```python
from build123d import *

# Parameters (mm, degrees)
EXTRUDE_1_DEPTH          = 129
CUT_EXTRUDE_1_DEPTH      = 131.732551417
CUT_EXTRUDE_1_DEPTH_BACK = 131.732551417
SKETCH_2_R               = 2.5
SKETCH_2_R_2             = 2


with BuildPart() as part:
    # 草图1 → 凸台-拉伸1 (new, symmetric)
    with BuildSketch(Plane(origin=(0, 0, 0), x_dir=(0, 0, -1), z_dir=(1, 0, 0))):
        with BuildLine():
            Line((-11, -15), (11, -15))
            ThreePointArc((11, -15), (13.828427125, -13.828427125), (15, -11))
            Line((15, -11), (15, 11))
            ThreePointArc((15, 11), (13.828427125, 13.828427125), (11, 15))
            Line((11, 15), (-11, 15))
            ThreePointArc((-11, 15), (-13.828427125, 13.828427125), (-15, 11))
            Line((-15, 11), (-15, -11))
            ThreePointArc((-15, -11), (-13.828427125, -13.828427125), (-11, -15))
        make_face()
        with BuildLine():
            Line((-11, -13), (11, -13))
            ThreePointArc((11, -13), (12.414213562, -12.414213562), (13, -11))
            Line((13, -11), (13, 11))
            ThreePointArc((13, 11), (12.414213562, 12.414213562), (11, 13))
            Line((11, 13), (-11, 13))
            ThreePointArc((-11, 13), (-12.414213562, 12.414213562), (-13, 11))
            Line((-13, 11), (-13, -11))
            ThreePointArc((-13, -11), (-12.414213562, -12.414213562), (-11, -13))
        make_face(mode=Mode.SUBTRACT)
    extrude(amount=EXTRUDE_1_DEPTH, both=True)

    # 草图2 → 切除-拉伸1 (cut, two sides: drawn at the far end of the back side and taken through both)
    with BuildSketch(Plane.XY.offset(-CUT_EXTRUDE_1_DEPTH_BACK)):
        with Locations((-75, -2.5)):
            Circle(SKETCH_2_R)
        with Locations(Location((75, -2.5, 0), (0, 0, 90))):
            Circle(SKETCH_2_R)
        with Locations((-65, -2.5)):
            Circle(SKETCH_2_R_2)
        with Locations(Location((65, -2.5, 0), (0, 0, 90))):
            Circle(SKETCH_2_R_2)
    extrude(amount=CUT_EXTRUDE_1_DEPTH + CUT_EXTRUDE_1_DEPTH_BACK, mode=Mode.SUBTRACT)


solid = part.part
```
Here's how the part is built. I have some questions about the finished solid (model axes, mm). A direction names the side the tool comes from. Give positions to 0.01 mm unless a question says otherwise; leave off trailing zeros. Loops run counter-clockwise (first coordinate to the right, second up) from the corner with the lowest first, then second, coordinate; pieces in that order, holes last. Notation, with made-up numbers: M -16,61 L -10,61 A20 ccw -10,80 Z; hole C -18.75,-23 d9. An arc over 180 degrees is marked long. Return JSON: item names as keys, results as strings.
Item 1: Thinking about a two-plate mould opening in X: for faces 3 (the flat face through (129, 0, 14)), 4 (the cylindrical face through (77, -1, 14)), 5 (the cylindrical face through (1.806, -13.797, 13.859)), which applies, released by +X, released by -X, zero draft, split by the parting line, or undercut?
A:
{"face 3": "released by +X", "face 4": "undercut", "face 5": "zero draft"}
Item 2: Imagine slicing it at A-A on x = 75. List the corners of the cut face in (y, z) for me.
A:
{"outline": "M -15,-11 A4 ccw -11,-15 L -5,-15 L -5,-13 L -11,-13 A2 cw -13,-11 L -13,11 A2 cw -11,13 L -5,13 L -5,15 L -11,15 A4 ccw -15,11 Z; M 0,-15 L 11,-15 A4 ccw 15,-11 L 15,11 A4 ccw 11,15 L 0,15 L 0,13 L 11,13 A2 cw 13,11 L 13,-11 A2 cw 11,-13 L 0,-13 Z"}
Item 3: Imagine slicing it at B-B on y = 6.5. List the corners of the cut face in (x, z) for me.
A:
{"outline": "M -129,-15 L 129,-15 L 129,-13 L -129,-13 Z; M -129,13 L 129,13 L 129,15 L -129,15 Z"}
Item 4: Imagine slicing it at D-D on x = 8.5. List the corners of the cut face in (y, z) for me.
A:
{"outline": "M -15,-11 A4 ccw -11,-15 L 11,-15 A4 ccw 15,-11 L 15,11 A4 ccw 11,15 L -11,15 A4 ccw -15,11 Z; hole M -13,-11 A2 ccw -11,-13 L 11,-13 A2 ccw 13,-11 L 13,11 A2 ccw 11,13 L -11,13 A2 ccw -13,11 Z"}
Item 5: On a 3-axis mill with a long thin cutter (end or side, diameter ignored), from which of +Z, -Z, +X, -X, +Y, -Y can I reach the whole of each face in a straight line? I mean faces 1 (the cylindrical face through (-63.153, -3.266, -14.014)), 2 (the flat face through (2, 0, 13)). Say none if no direction works.
A:
{"face 1": "+Z, -Z", "face 2": "+X, -X"}
Item 6: Please list where these lines run through material, in increasing order: line 1 (X direction, y = -2.5, z = 14.4); line 2 (Z direction, x = -112, y = -1.25).
A:
{"line 1": "x = -129 to -77.5, -72.5 to -67, -63 to 63, 67 to 72.5, 77.5 to 129", "line 2": "z = -15 to -13, 13 to 15"}
